Could you check a few things on this model? Use its own coordinates, in mm. Face numbers are marked on the shaded views. Coordinates: 2 decimals unless noted, no trailing zeros. Write each loop counter-clockwise with the first axis right and the second up, starting at its lowest first coordinate (ties: lowest second). Pieces come first, ordered by that corner, then holes.
Item 1: I want a section at A-A on x = 0. Please give me the cut outline in (y, z), then the cut area to 3 significant figures.
Item 2: If I drill on probe 1 along Y at (x, z) = (-1, 55.5); probe 2 along X at (y, z) = (0.5, 94); probe 3 along Y at (x, z) = (0, 75.5), over which ranges is the centre line in solid material (lowest first)?
Item 3: For P1, Ø6, axis at x = 7, y = -7, coming from the +Z side; P2, Ø1.5, axis at x = 15, z = 52.5, coming from the +Y side; P3, Ø12, axis at x = 22.5, z = 58, coming from the -Y side, each with a flat end and sliding along its axis, tell me the tip position at first contact or that it passes through.
Item 4: I want a section at D-D on y = 26. Please give me the cut outline in (x, z).
Item 5: Thinking about a two-plate mould opening in X: for the marked faces 1, 2 and 3, which applies, +X half, -X half, draft (parallel to the pull), parting line (faces both ways), or undercut?
Item 6: I want a section at C-C on z = 60.5. Please give me the cut outline in (x, y).
Item 7: I want a section at B-B on y = 0. Please give me the cut outline in (x, z), then the cut area to 3 significant figures.
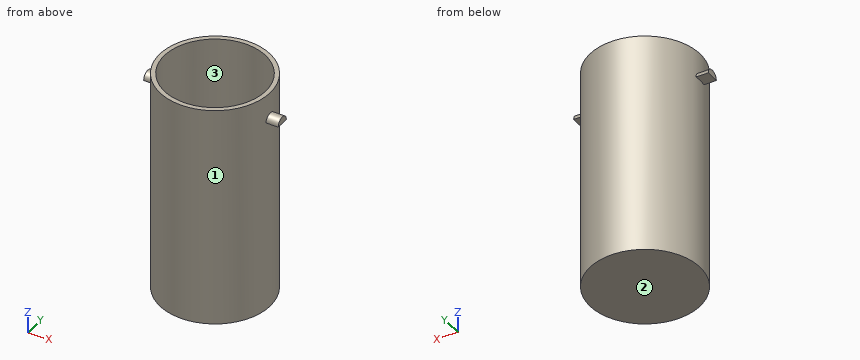
from build123d import *

# Parameters (mm, degrees)
SKETCH1_R                = 31.369
BOSS_EXTRUDE1_DEPTH      = 127
BOSS_EXTRUDE2_DEPTH      = 38.1
BOSS_EXTRUDE2_DEPTH_BACK = 38.1
SHELL3_START             = 2.54
SHELL3_OUTLINE_R         = 28.829
SHELL3_DEPTH             = 124.46


# Read off the part's stored shape, not the designer's step: Shell3
with BuildPart() as part:
    # Sketch1 → Boss-Extrude1 (new body)
    with BuildSketch(Plane.XY):
        Circle(SKETCH1_R)
    extrude(amount=BOSS_EXTRUDE1_DEPTH)

    # Sketch2 → Boss-Extrude2 (add, two sides: drawn at the far end of the back side and taken through both)
    with BuildSketch(Plane(origin=(0, 0, 0), x_dir=(0, 0, -1), z_dir=(1, 0, 0)).offset(-BOSS_EXTRUDE2_DEPTH_BACK)):
        with BuildLine():
            Line((-111.161571782, 3.81), (-111.161571782, -3.81))
            ThreePointArc((-111.161571782, -3.81), (-114.971571782, 0), (-111.161571782, 3.81))
        make_face()
    extrude(amount=BOSS_EXTRUDE2_DEPTH + BOSS_EXTRUDE2_DEPTH_BACK)

    # Shell3 outline → Shell3 (cut)
    with BuildSketch(Plane.XY.offset(SHELL3_START)):
        Circle(SHELL3_OUTLINE_R)
    extrude(amount=SHELL3_DEPTH, mode=Mode.SUBTRACT)


solid = part.part
Response values:
1. outline: (-31.37, 0) - (31.37, 0) - (31.37, 127) - (28.83, 127) - (28.83, 2.54) - (-28.83, 2.54) - (-28.83, 127) - (-31.37, 127) - close
1. area: 792 mm2
2. probe 1: y = -31.35 to -28.81, 28.81 to 31.35
2. probe 2: x = -31.37 to -28.82, 28.82 to 31.37
2. probe 3: y = -31.37 to -28.83, 28.83 to 31.37
3. P1: stops at z = 2.54
3. P2: stops at y = 27.95
3. P3: stops at y = -26.68
4. outline: (-17.55, 0) - (17.55, 0) - (17.55, 127) - (12.45, 127) - (12.45, 2.54) - (-12.45, 2.54) - (-12.45, 127) - (-17.55, 127) - close
5. face 1: parting line
5. face 2: draft
5. face 3: undercut
6. outline: circle Ø62.74 at (0, 0); hole circle Ø57.66 at (0, 0)
7. outline: (-38.1, 111.16) - (-31.37, 111.16) - (-31.37, 0) - (31.37, 0) - (31.37, 111.16) - (38.1, 111.16) - (38.1, 114.97) - (31.37, 114.97) - (31.37, 127) - (28.83, 127) - (28.83, 2.54) - (-28.83, 2.54) - (-28.83, 127) - (-31.37, 127) - (-31.37, 114.97) - (-38.1, 114.97) - close
7. area: 843 mm2
